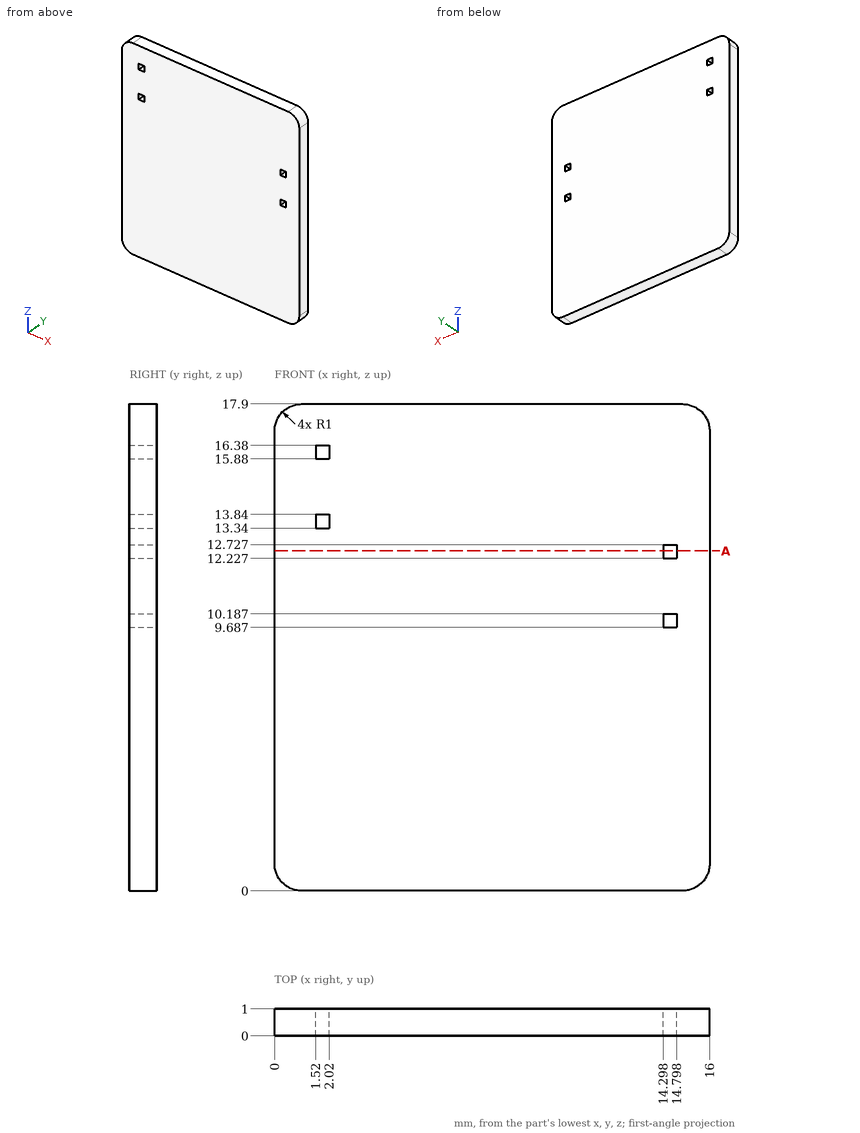
Here's the drawing with two shaded views (mm, measured from the low corner). I have some questions. Coordinates: 2 decimals unless noted, no trailing zeros. Write each loop counter-clockwise with the first axis right and the second up, starting at its lowest first coordinate (ties: lowest second). Pieces come first, ordered by that corner, then holes. Notation, with made-up numbers: (67, 73) - (97, 73) arc R32 cw to (97, 112) - close; hole circle Ø10 at (-22.5, -4.75). An arc over 180 degrees is marked (long way). Return JSON: item names as keys, results as strings.
Q1. I'm going to push a flat-ended pin straight in: pin 1 Ø0.6 at (y, z) = (0.5, 12.5) entering from -X. Where does the tip first touch, or does it pass through?
Computed values:
{"pin 1": "stops at x = 0"}
Q2. If we section it at A-A (z = 12.5): Please give me the cut outline in (x, y), then the cut area to 3 significant figures.
Computed values:
{"outline": "(0, 0) - (14.3, 0) - (14.3, 1) - (0, 1) - close; (14.8, 0) - (16, 0) - (16, 1) - (14.8, 1) - close", "area": "15.5 mm2"}
Q3. Please list where these lines run through material, in increasing order: L1, parallel to Z at x = 14.5, y = 0.45; L2, parallel to X at y = 0.15, z = 13.5; L3, parallel to X at y = 0.55, z = 17. Write a range as from..to.
Computed values:
{"L1": "z = 0..9.69, 10.19..12.23, 12.73..17.9", "L2": "x = 0..1.52, 2.02..16", "L3": "x = 0.01..15.99"}
